Work out the finished part from the listing and answer in its coordinate system (mm). A direction names the side the tool comes from. Give positions to 0.01 mm unless a question says otherwise; leave off trailing zeros. Loops run counter-clockwise (first coordinate to the right, second up) from the corner with the lowest first, then second, coordinate; pieces in that order, holes last. Notation, with made-up numbers: M 37.25,15.25 L 54.25,15.25 A13 ccw 54.25,34.25 Z; hole C 21,74 d2. An arc over 180 degrees is marked long. Answer as a JSON object with one key per item and string values. Group by question number.
```python
from build123d import *

# Parameters (mm, degrees)
SKETCH1_W           = 3.4163
SKETCH1_H           = 6.477
EXTRUDE1_DEPTH      = 3.8354
SKETCH2_W           = 0.5588
SKETCH2_H           = 6.477
EXTRUDE2_DEPTH      = 0.3048
SKETCH3_W           = 4.5212
SKETCH3_H           = 8.255
EXTRUDE3_DEPTH      = 1.016
SKETCH4_W           = 2.4638
SKETCH4_H           = 2.4638
SKETCH4_W_2         = 1.4478
SKETCH4_H_2         = 1.4478
EXTRUDE4_DEPTH      = 6.2738
SKETCH5_W           = 2.4638
SKETCH5_H           = 2.5146
EXTRUDE5_DEPTH      = 7.2898
EXTRUDE6_DEPTH      = 2.4765
EXTRUDE6_DEPTH_BACK = 2.4765


with BuildPart() as part:
    # Sketch1 → Extrude1 (new body)
    with BuildSketch(Plane.XY):
        with Locations((1.70815, 3.2385)):
            Rectangle(SKETCH1_W, SKETCH1_H)
    extrude1 = extrude(amount=EXTRUDE1_DEPTH)

    # Mirror1: Extrude1 across plane
    add(extrude1.mirror(Plane.XY.offset(3.8354)))

    # Sketch2 → Extrude2 (add)
    with BuildSketch(Plane(origin=(3.4163, 0, 0), x_dir=(0, 0, -1), z_dir=(1, 0, 0))):
        with Locations((-5.7404, 3.2385)):
            Rectangle(SKETCH2_W, SKETCH2_H)
    extrude(amount=EXTRUDE2_DEPTH)

    # Sketch3 → Extrude3 (add)
    with BuildSketch(Plane.XZ):
        with Locations((2.2606, 3.8354)):
            Rectangle(SKETCH3_W, SKETCH3_H)
    extrude(amount=EXTRUDE3_DEPTH)

    # Sketch4 → Extrude4 (add)
    # profile 1 of 2: a face of its own
    with BuildSketch(Plane(origin=(0, 6.477, 0), x_dir=(1, 0, 0), z_dir=(0, 1, 0))):
        Polygon((2.9464, -6.6294), (0.4826, -6.6294), (0.4826, -4.1656), (2.084295412, -4.1656), (2.9464, -5.027704588), align=None)
        Polygon((0.9906, -6.1214), (0.9906, -4.6736), (1.873874923, -4.6736), (2.4384, -5.238125077), (2.4384, -6.1214), align=None, mode=Mode.SUBTRACT)
    # profile 2 of 2: a face of its own
    with BuildSketch(Plane(origin=(0, 6.477, 0), x_dir=(1, 0, 0), z_dir=(0, 1, 0))):
        with Locations((1.7145, -2.2733)):
            Rectangle(SKETCH4_W, SKETCH4_H)
        with Locations((1.7145, -2.2733)):
            Rectangle(SKETCH4_W_2, SKETCH4_H_2, mode=Mode.SUBTRACT)
    extrude(amount=EXTRUDE4_DEPTH)

    # Sketch5 → Extrude5 (cut)
    with BuildSketch(Plane.XZ.offset(1.016)):
        with Locations((1.8669, 5.3086)):
            Rectangle(SKETCH5_W, SKETCH5_H)
        with Locations((1.8669, 2.3622)):
            Rectangle(SKETCH5_W, SKETCH5_H)
    extrude(amount=-EXTRUDE5_DEPTH, mode=Mode.SUBTRACT)

    # Sketch6 → Extrude6 (add, two sides: drawn at the far end of the back side and taken through both)
    with BuildSketch(Plane.XY.offset(3.8354).offset(-EXTRUDE6_DEPTH_BACK)):
        with BuildLine():
            ThreePointArc((-0.6096, 0.7874), (-0.617039488, 0.769439488), (-0.635, 0.762))
            Line((-0.635, 0.762), (-2.0574, 0.762))
            ThreePointArc((-2.0574, 0.762), (-2.075360512, 0.769439488), (-2.0828, 0.7874))
            Line((-2.0828, 0.7874), (-2.0828, 2.0066))
            ThreePointArc((-2.0828, 2.0066), (-2.075360512, 2.024560512), (-2.0574, 2.032))
            Line((-2.0574, 2.032), (-1.8034, 2.032))
            ThreePointArc((-1.8034, 2.032), (-1.785439488, 2.039439488), (-1.778, 2.0574))
            Line((-1.778, 2.0574), (-1.778, 4.6736))
            ThreePointArc((-1.778, 4.6736), (-1.770560512, 4.691560512), (-1.7526, 4.699))
            Line((-1.7526, 4.699), (-1.549059076, 4.699))
            ThreePointArc((-1.549059076, 4.699), (-1.53122032, 4.706318551), (-1.523661395, 4.724056788))
            Line((-1.523661395, 4.724056788), (-1.424588234, 12.055470697))
            ThreePointArc((-1.424588234, 12.055470697), (-1.403642896, 12.080134217), (-1.375472083, 12.06421562))
            Line((-1.375472083, 12.06421562), (-0.61128153, 10.069809609))
            ThreePointArc((-0.61128153, 10.069809609), (-0.61002392, 10.065342668), (-0.6096, 10.060721474))
            Line((-0.6096, 10.060721474), (-0.6096, 5.882065653))
            ThreePointArc((-0.6096, 5.882065653), (-0.602160512, 5.864105141), (-0.5842, 5.856665653))
            Line((-0.5842, 5.856665653), (0, 5.856665653))
            Line((0, 5.856665653), (0, 4.434265653))
            Line((0, 4.434265653), (-0.5842, 4.434265653))
            ThreePointArc((-0.5842, 4.434265653), (-0.602160512, 4.426826165), (-0.6096, 4.408865653))
            Line((-0.6096, 4.408865653), (-0.6096, 0.7874))
        make_face()
    extrude(amount=EXTRUDE6_DEPTH + EXTRUDE6_DEPTH_BACK)


solid = part.part
```
Item 1: Given pin 1 Ø3 at (x, y) = (4, 4) entering from +Z; pin 2 Ø2 at (x, y) = (1.5, 11) entering from -Z; pin 3 Ø1.2 at (x, y) = (2, 3) entering from -Z, each flat-ended and moving along its own axis, determine where each tip first touches the part or whether it passes through.
Item 2: Find the intervals of material crossed by probe 1 along Z at (x, y) = (1, 4.75); probe 2 along X at (y, z) = (5.75, 6.5) (3 decimals); probe 3 along X at (y, z) = (1, 2.25) (3 decimals), in increasing order. Write a range as [from, to].
Item 3: A tool of negligible diameter and unlimited length cuts with its end or side. For faces 1 (the flat face through (2, 3, 0)), 2 (the flat face through (2.946, 10, 2)), 3 (the flat face through (1, 10, 4.166)), from which of +Z, -Z, +X, -X, +Y, -Y can it reach the whole face along a straight path? Write none if from no direction.
Item 4: For a pull along X with two mould halves and no side action, classify faces 4 (the flat face through (-1, 5, 6.312)), 5 (the flat face through (2.946, 10, 6)), 6 (the flat face through (0.635, 3, 2)) as pulls with the +X half, pulls with the -X half, needs draft (parallel to the pull), parting line crosses it, or undercut.
Item 5: A cutting plane is placed at A-A (y = 3.5). Give the number of separate pieces and of enclosed holes in the cut face, and give its area (3 significant figures).
Item 6: A cutting plane is placed at B-B (y = 9.5). Determine the outline of the cut face in (x, z).
Item 7: A cutting plane is placed at C-C (x = 0.25). Determine the outline of the cut face in (y, z), and give its area (3 significant figures).
The answers:
{
 "1": {"pin 1": "stops at z = 7.67", "pin 2": "stops at z = 1.04", "pin 3": "stops at z = 0"},
 "2": {"probe 1": "z = [0, 1.1], [3.62, 4.05], [6.57, 7.67]", "probe 2": "x = [0, 0.635], [3.099, 3.416]", "probe 3": "x = [-2.083, -0.61], [0, 0.635], [3.099, 3.416]"},
 "3": {"face 1": "-Z, +X, -X, +Y", "face 2": "+Z, -Z, +X, +Y", "face 3": "+X, +Y"},
 "4": {"face 4": "needs draft", "face 5": "pulls with the +X half", "face 6": "undercut"},
 "5": {"separate pieces": "2", "enclosed holes": "2", "area": "19.8 mm^2"},
 "6": {"outline": "M -1.46,1.36 L -0.61,1.36 L -0.61,6.31 L -1.46,6.31 Z; M 0.48,1.04 L 2.95,1.04 L 2.95,3.51 L 0.48,3.51 Z; M 0.48,4.17 L 2.08,4.17 L 2.95,5.03 L 2.95,6.63 L 0.48,6.63 Z; hole M 0.99,1.55 L 2.44,1.55 L 2.44,3 L 0.99,3 Z; hole M 0.99,4.67 L 1.87,4.67 L 2.44,5.24 L 2.44,6.12 L 0.99,6.12 Z"},
 "7": {"outline": "M -1.02,-0.29 L 0,-0.29 L 0,0 L 6.48,0 L 6.48,7.67 L 0,7.67 L 0,7.96 L -1.02,7.96 Z", "area": "58.1 mm^2"}
}
